For this review, use the dimensioned drawing (mm, ordinates from the lowest corner) and the shaded views. Give positions to 0.01 mm unless a question says otherwise; leave off trailing zeros. Write each loop counter-clockwise with the first axis right and the second up, starting at its lowest first coordinate (ties: lowest second). Pieces come first, ordered by that corner, then holes. Notation, with made-up numbers: M 65,48 L 122,48 A32 ccw 122,83 Z; hole C 40,68 d6. An arc over 180 degrees is marked long. Answer in a Markdown table with one row per item.
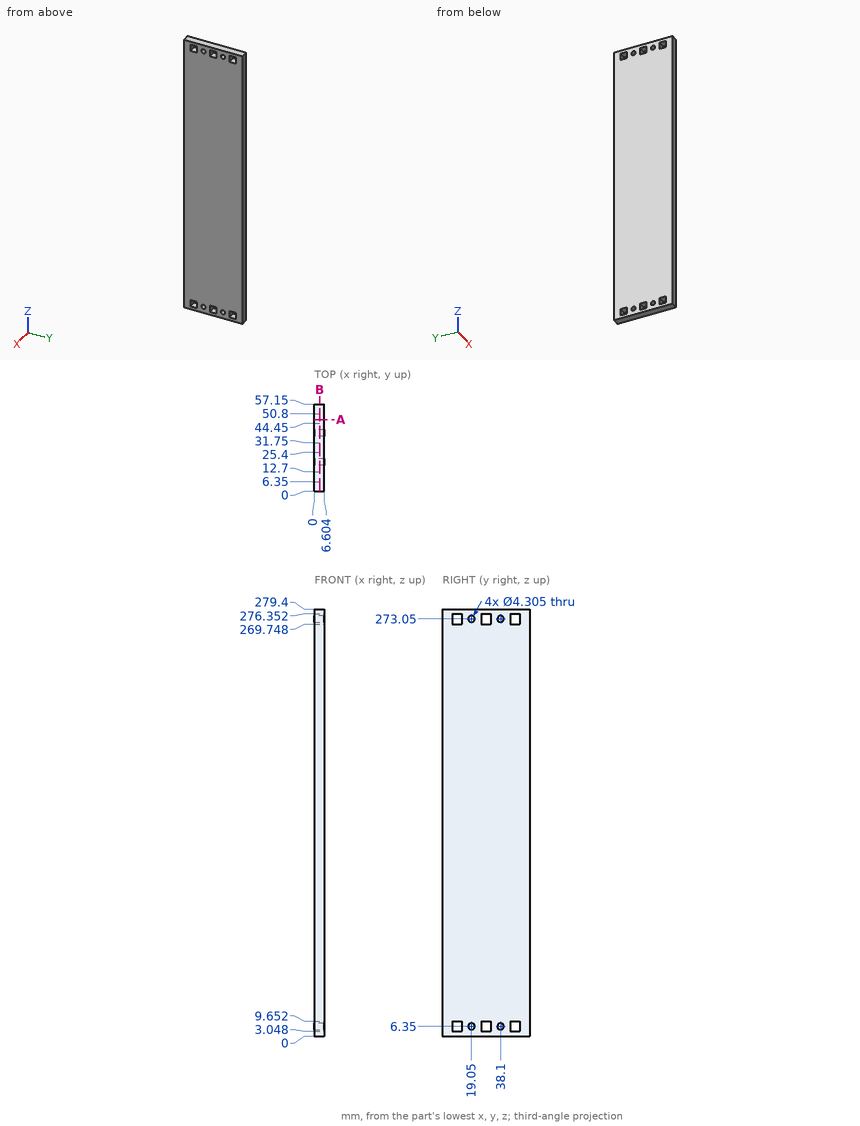
1) To check wall thickness, follow probe 1 along Y at (x, z) = (2.5, 6.35); probe 2 along Z at (x, y) = (1.25, 19); probe 3 along Z at (x, y) = (3.25, 27). State the ranges of each line that lie inside material, in increasing order. Write a range as [from, to].
Geometry says:
| item | result |
|---|---|
| probe 1 | [0, 6.35], [12.7, 16.9], [21.2, 25.4], [31.75, 35.95], [40.25, 44.45], [50.8, 57.15] |
| probe 2 | [0, 4.2], [8.5, 270.9], [275.2, 279.4] |
| probe 3 | [0, 3.05], [9.65, 269.75], [276.35, 279.4] |
2) Insertion check: P1, Ø2.5, axis at y = 38.1, z = 6.35, coming from the -X side. The pin has a flat end and moves straight along its axis. Give the tip position at first contact, or say it passes through.
Geometry says:
| item | result |
|---|---|
| P1 | through |
3) Add section A-A (y = 47). Write out the cut boundary in (x, z), and give its area (3 significant figures).
Geometry says:
| item | result |
|---|---|
| outline | M 0,0 L 6.6,0 L 6.6,3.05 L 0,3.05 Z; M 0,9.65 L 6.6,9.65 L 6.6,269.75 L 0,269.75 Z; M 0,276.35 L 6.6,276.35 L 6.6,279.4 L 0,279.4 Z |
| area | 1,760 mm^2 |
4) Add section B-B (x = 3.5). Count the separate pieces of the cut face and the enclosed holes in it, and give its area (3 significant figures).
Geometry says:
| item | result |
|---|---|
| separate pieces | 1 |
| enclosed holes | 10 |
| area | 15,700 mm^2 |
